Could you check a few things on this model? Use its own coordinates, in mm. A direction names the side the tool comes from. Give positions to 0.01 mm unless a question says otherwise; leave off trailing zeros. Write each loop counter-clockwise with the first axis right and the second up, starting at its lowest first coordinate (ties: lowest second). Pieces come first, ordered by that corner, then holes. Notation, with made-up numbers: (55.5, -29.75) - (79.5, -29.75) arc R22 ccw to (79.5, -13.75) - close; hole circle Ø4 at (46.25, 87.25). An arc over 180 degrees is marked (long way). Answer in a Markdown table with one row per item.
from build123d import *

# Parameters (mm, degrees)
SKETCH2_R           = 0.3
BOSS_EXTRUDE1_DEPTH = 2.54


with BuildPart() as part:
    # Sketch1 → Revolve1 (revolve)
    with BuildSketch(Plane.XY, mode=Mode.PRIVATE) as revolve1_sk:
        with BuildLine():
            Line((2.5, 7.1), (2.5, 1))
            Line((2.5, 1), (3.148870311, 1))
            Line((3.148870311, 1), (3.148870311, 0))
            Line((3.148870311, 0), (0, 0))
            Line((0, 0), (0, 7.1))
            Line((0, 7.1), (0, 9.6))
            ThreePointArc((0, 9.6), (1.767766953, 8.867766953), (2.5, 7.1))
        make_face()
    revolve(revolve1_sk.sketch.rotate(Axis((0, 7.1, 0), (0, -1, 0)), 90), axis=Axis((0, 7.1, 0), (0, -1, 0)))

    # Sketch2 → Boss-Extrude1 (add)
    with BuildSketch(Plane.XZ):
        with Locations(Location((-1.27, 0, 0), (0, 0, 90))):
            Circle(SKETCH2_R)
        with Locations(Location((1.27, 0, 0), (0, 0, 90))):
            Circle(SKETCH2_R)
    extrude(amount=BOSS_EXTRUDE1_DEPTH)


solid = part.part
1) Imagine slicing it at A-A (x = 0). List the corners of the cut face in (y, z) for me.
Check values:
| item | result |
|---|---|
| outline | (0, -3.15) - (1, -3.15) - (1, -2.5) - (7.1, -2.5) arc R2.5 ccw to (7.1, 2.5) - (1, 2.5) - (1, 3.15) - (0, 3.15) - close |
2) Imagine slicing it at D-D (z = 1.25). List the corners of the cut face in (x, y) for me.
Check values:
| item | result |
|---|---|
| outline | (-2.89, 0) - (2.89, 0) - (2.89, 1) - (2.17, 1) - (2.17, 7.1) arc R2.17 ccw to (-2.17, 7.1) - (-2.17, 1) - (-2.89, 1) - close |
3) On a 3-axis mill with a long thin cutter (end or side, diameter ignored), from which of +Z, -Z, +X, -X, +Y, -Y can I reach the whole of each face in a straight line? I mean faces 1 (the face through (-3.122, 0.493, -0.41)), 2 (the face through (-0.1, 4, -2.5)). Say none if no direction works.
Check values:
| item | result |
|---|---|
| face 1 | +Y, -Y |
| face 2 | +Y |
4) If I drill on line 1 (Y direction, x = 0.5, z = -2.5); line 2 (X direction, y = 4.5, z = 1.5); line 3 (X direction, y = 4.75, z = 0.5), over which ranges is the centre line in solid material (lowest first)?
Check values:
| item | result |
|---|---|
| line 1 | y = 0 to 1 |
| line 2 | x = -2 to 2 |
| line 3 | x = -2.45 to 2.45 |
5) Will these pins go through, and if not, where does the flat tip stop? P1, Ø1.9, axis at x = -1.5, z = 1, coming from the +Y side; P2, Ø1.5, axis at y = 5, z = 0.5, coming from the +X side; P3, Ø2, axis at y = 3.5, z = 0.5, coming from the -X side.
Check values:
| item | result |
|---|---|
| P1 | stops at y = 9.45 |
| P2 | stops at x = 2.5 |
| P3 | stops at x = -2.5 |
6) Imagine slicing it at B-B (z = 0). List the corners of the cut face in (x, y) for me, then the cut area to 3 significant figures.
Check values:
| item | result |
|---|---|
| outline | (-3.15, 0) - (-1.57, 0) - (-1.57, -2.54) - (-0.97, -2.54) - (-0.97, 0) - (0.97, 0) - (0.97, -2.54) - (1.57, -2.54) - (1.57, 0) - (3.15, 0) - (3.15, 1) - (2.5, 1) - (2.5, 7.1) arc R2.5 ccw to (-2.5, 7.1) - (-2.5, 1) - (-3.15, 1) - close |
| area | 49.7 mm2 |
7) Imagine slicing it at C-C (y = 5.75). List the corners of the cut face in (x, z) for me, then the cut area to 3 significant figures.
Check values:
| item | result |
|---|---|
| outline | circle Ø5 at (0, 0) |
| area | 19.6 mm2 |
